from build123d import *

# Parameters (mm, degrees)
F0_R      = 30
F1_DEPTH  = 9
F2_R      = 25.25
F3_DEPTH  = 4
F4_R      = 1.5
F5_DEPTH  = 9.001
F6_R      = 1.35
F7_DEPTH  = 9.001
F8_R      = 2.75
F9_DEPTH  = 5.001
F10_R     = 30
F10_R_2   = 20
F11_DEPTH = 5
F12_W     = 30
F12_H     = 24.764763
F13_DEPTH = 5


with BuildPart() as f1:
    # F0 (on Top) → F1 (new body)
    with BuildSketch(Plane.XY):
        Circle(F0_R)
    extrude(amount=F1_DEPTH)

    # F2 (on face) → F3 (cut)
    with BuildSketch(Plane.XY.offset(9)):
        Circle(F2_R)
    extrude(amount=-F3_DEPTH, mode=Mode.SUBTRACT)

    # F4 (on Top) → F5 (cut, through all)
    with BuildSketch(Plane.XY):
        Circle(F4_R)
    extrude(amount=F5_DEPTH, mode=Mode.SUBTRACT)

    # F6 (on face) → F7 (cut, through all)
    with BuildSketch(Plane.XY.offset(9)):
        with Locations((23.815699, 13.75)):
            Circle(F6_R)
        with Locations((0, -27.5)):
            Circle(F6_R)
        with Locations((-23.815699, 13.75)):
            Circle(F6_R)
    extrude(amount=-F7_DEPTH, mode=Mode.SUBTRACT)

    # F8 (on face) → F9 (cut, through all)
    with BuildSketch(Plane.XY.offset(5)):
        with Locations((0, 17)):
            Circle(F8_R)
    extrude(amount=-F9_DEPTH, mode=Mode.SUBTRACT)

    # F10 (on face) → F11 (join)
    with BuildSketch(Plane(origin=(0, 0, 0), x_dir=(1, 0, 0), z_dir=(0, 0, -1))):
        Circle(F10_R)
        Circle(F10_R_2, mode=Mode.SUBTRACT)
    extrude(amount=F11_DEPTH)

    # F12 (on Top) → F13 (cut)
    with BuildSketch(Plane.XY):
        with Locations((0, 20.9111)):
            Rectangle(F12_W, F12_H)
    extrude(amount=-F13_DEPTH, mode=Mode.SUBTRACT)


solid = f1.part
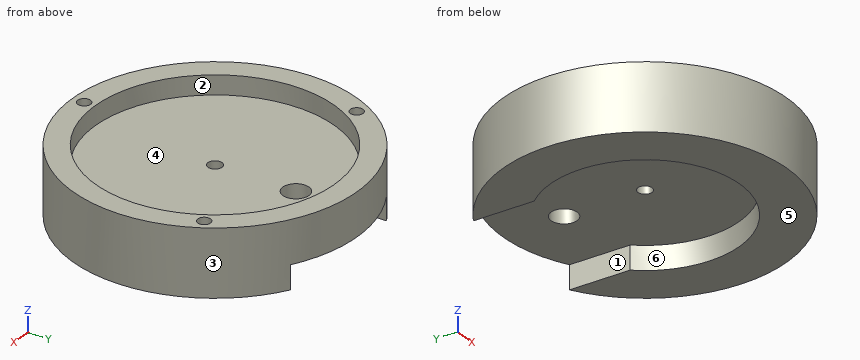
Geometry: final body of the model. Coordinates: model frame, mm. Face numbers are marked on the shaded views. A direction names the side the tool comes from. Give positions to 0.01 mm unless a question says otherwise; leave off trailing zeros. Write each loop counter-clockwise with the first axis right and the second up, starting at its lowest first coordinate (ties: lowest second). Pieces come first, ordered by that corner, then holes. Notation, with made-up numbers: (70, 2.25) -> (125, 2.25) arc R14 cw to (125, 11.25) -> close; hole circle Ø11 at (69, 21). An arc over 180 degrees is marked (long way). Answer in a Markdown table with one row per item.
(1) Section query C-C on z = 3. Return loops of the section in (x, y), then the cut area to 3 significant figures.
Answers below:
| item | result |
|---|---|
| outline | circle Ø60 at (0, 0); hole circle Ø2.7 at (-23.82, 13.75); hole circle Ø5.5 at (0, 17); hole circle Ø3 at (0, 0); hole circle Ø2.7 at (0, -27.5); hole circle Ø2.7 at (23.82, 13.75) |
| area | 2,780 mm^2 |
(2) Ray query, line 1 along Y through (x, z) = (0, 3.7); line 2 along Z through (x, y) = (-7, -24); line 3 along X through (y, z) = (0, -2.4). Return the intervals inside material, ascending. Write a range as [from, to].
Answers below:
| item | result |
|---|---|
| line 1 | [-30, -28.85], [-26.15, -1.5], [1.5, 14.25], [19.75, 30] |
| line 2 | [-5, 5] |
| line 3 | [-30, -20], [20, 30] |
(3) Draft query along Y for the marked faces 1, 2 and 3. Return one class per face: +Y half, -Y half, draft (parallel to the pull), parting line (faces both ways), or undercut.
Answers below:
| item | result |
|---|---|
| face 1 | draft |
| face 2 | undercut |
| face 3 | parting line |
(4) Set-up query: the marked faces 4, 5 and 6. Return all of +Z, -Z, +X, -X, +Y, -Y with unobstructed straight access to the full face (end or side cutting, diameter ignored); none if empty.
Answers below:
| item | result |
|---|---|
| face 4 | +Z |
| face 5 | -Z, +X, -X, +Y, -Y |
| face 6 | -Z |
(5) Pin query (flat end, axial travel): pin 1 (3 mm diameter, centred on x = 4.5, y = 20.5, fed in from +Z); pin 2 (2.5 mm diameter, centred on y = 19.5, z = -3, fed in from -X); pin 3 (1.3 mm diameter, centred on x = -23.5, y = 14, fed in from +Z). Return the tip coordinate at first contact, or that it passes through.
Answers below:
| item | result |
|---|---|
| pin 1 | z = 5 |
| pin 2 | x = -23.81 |
| pin 3 | z = 0 |
(6) Section query B-B on x = 0. Return loops of the section in (y, z).
Answers below:
| item | result |
|---|---|
| outline | (-30, -5) -> (-20, -5) -> (-20, 0) -> (-1.5, 0) -> (-1.5, 5) -> (-25.25, 5) -> (-25.25, 9) -> (-26.15, 9) -> (-26.15, 0) -> (-28.85, 0) -> (-28.85, 9) -> (-30, 9) -> close; (1.5, 0) -> (14.25, 0) -> (14.25, 5) -> (1.5, 5) -> close; (19.75, 0) -> (30, 0) -> (30, 9) -> (25.25, 9) -> (25.25, 5) -> (19.75, 5) -> close |
(7) Section query D-D on z = 6.5. Return loops of the section in (x, y).
Answers below:
| item | result |
|---|---|
| outline | circle Ø60 at (0, 0); hole circle Ø50.5 at (0, 0); hole circle Ø2.7 at (-23.82, 13.75); hole circle Ø2.7 at (0, -27.5); hole circle Ø2.7 at (23.82, 13.75) |
(8) Section query A-A on y = 0. Return loops of the section in (x, z).
Answers below:
| item | result |
|---|---|
| outline | (-30, -5) -> (-20, -5) -> (-20, 0) -> (-1.5, 0) -> (-1.5, 5) -> (-25.25, 5) -> (-25.25, 9) -> (-30, 9) -> close; (1.5, 0) -> (20, 0) -> (20, -5) -> (30, -5) -> (30, 9) -> (25.25, 9) -> (25.25, 5) -> (1.5, 5) -> close |
